```python
from build123d import *

# Parameters (mm, degrees)
F0_W      = 4.7625
F0_H      = 457.2
F1_DEPTH  = 609.6
F2_W      = 50.8
F2_H      = 4.7625
F3_DEPTH  = 609.6
F4_DEPTH  = 609.6
F5_W      = 25.4
F5_H      = 461.9625
F6_DEPTH  = 25.4
F8_DEPTH  = 25.4
F9_W      = 1637.8936
F9_H      = 25.4
F10_DEPTH = 25.4
F11_W     = 25.4
F11_H     = 433.81924
F12_DEPTH = 25.4
F13_DEPTH = 25.4
F14_W     = 25.4
F14_H     = 432.793116
F15_DEPTH = 25.4
F16_W     = 1636.5474
F16_H     = 25.4
F17_DEPTH = 25.4
F18_W     = 25.4
F18_H     = 609.6
F19_DEPTH = 25.4
F20_W     = 50.8
F20_H     = 453.430616
F21_DEPTH = 4.7625
F22_W     = 25.4
F22_H     = 457.2
F23_DEPTH = 4.7625


with BuildPart() as f1:
    # F0 (on Front) → F1 (new body)
    with BuildSketch(Plane.XZ):
        with Locations((-455.648437, -32.960023)):
            Rectangle(F0_W, F0_H)
        Polygon((-415.167187, -261.560023), (-453.267187, -261.560023), (-458.029687, -261.560023), (-458.029687, -266.322523), (-415.167187, -266.981946), align=None)
        Polygon((-408.817187, 151.189977), (-415.167187, -261.560023), (-415.167187, -266.981946), (-410.404687, -266.981946), (-404.044542, 146.427477), (-408.817187, 146.427477), align=None)
        Polygon((-403.971273, 151.189977), (-408.817187, 151.189977), (-408.817187, 146.427477), (-404.044542, 146.427477), align=None)
        Polygon((286.507813, 151.189977), (-403.971273, 151.189977), (-404.044542, 146.427477), (281.781948, 146.427477), (286.544448, 146.427477), align=None)
        Polygon((289.682813, -261.560023), (286.544448, 146.427477), (281.781948, 146.427477), (284.920313, -261.560023), align=None)
        Polygon((327.782813, -261.560023), (289.682813, -261.560023), (284.920313, -261.560023), (284.920313, -266.322523), (327.782813, -266.322523), align=None)
        Polygon((330.957813, 151.189977), (327.782813, -261.560023), (327.782813, -266.322523), (332.545172, -266.359156), (335.720454, 146.427477), (330.957813, 146.427477), align=None)
        Polygon((335.757089, 151.189977), (330.957813, 151.189977), (330.957813, 146.427477), (335.720454, 146.427477), align=None)
        Polygon((1021.520313, 151.189977), (335.757089, 151.189977), (335.720454, 146.427477), (1021.593582, 146.427477), align=None)
        Polygon((1026.282813, 151.189977), (1021.520313, 151.189977), (1021.593582, 146.427477), (1026.356082, 146.427477), align=None)
        Polygon((1026.356082, 146.427477), (1021.593582, 146.427477), (1027.870313, -261.560023), (1032.632813, -261.560023), align=None)
        Polygon((1032.632813, -261.560023), (1027.870313, -261.560023), (1027.870313, -266.322523), (1070.732813, -266.322523), (1070.732813, -261.560023), align=None)
        Polygon((1070.732813, 190.877477), (1070.732813, -261.560023), (1070.732813, -266.322523), (1075.495313, -266.322523), (1075.495313, 190.877477), align=None)
    extrude(amount=-F1_DEPTH)

    # F2 (on face) → F3 (join)
    with BuildSketch(Plane.XZ):
        with Locations((-483.429687, 193.258727)):
            Rectangle(F2_W, F2_H)
    extrude(amount=-F3_DEPTH)

    # F2 (on face) → F4 (join)
    with BuildSketch(Plane.XZ):
        with Locations((-483.429687, 193.258727)):
            Rectangle(F2_W, F2_H)
        with Locations((1100.895313, 188.496227)):
            Rectangle(F2_W, F2_H)
    extrude(amount=-F4_DEPTH)

    # F5 (on face) → F6 (join)
    with BuildSketch(Plane.XZ):
        with Locations((-496.129687, -40.103773)):
            Rectangle(F5_W, F5_H)
        with Locations((1113.595313, -44.866273)):
            Rectangle(F5_W, F5_H)
    extrude(amount=-F6_DEPTH)

    # F5 (on face) → F8 (join)
    with BuildSketch(Plane.XZ):
        with Locations((-496.129687, -40.103773)):
            Rectangle(F5_W, F5_H)
        with Locations((1113.595313, -44.866273)):
            Rectangle(F5_W, F5_H)
    extrude(amount=-F8_DEPTH)

    # F9 (on face) → F10 (join)
    with BuildSketch(Plane.XZ):
        with Locations((308.156171, -281.041763)):
            Rectangle(F9_W, F9_H)
    extrude(amount=-F10_DEPTH)

    # F11 (on face) → F12 (join)
    with BuildSketch(Plane.YZ.offset(1126.295313)):
        Polygon((609.6, 190.877477), (0, 190.877477), (0, 165.477477), (584.2, 165.477477), (609.6, 165.477477), align=None)
        with Locations((596.9, -51.432143)):
            Rectangle(F11_W, F11_H)
        Polygon((609.6, -293.741763), (609.6, -268.341763), (584.2, -268.341763), (25.4, -268.341763), (25.4, -293.741763), align=None)
    extrude(amount=-F12_DEPTH)

    # F11 (on face) → F13 (join)
    with BuildSketch(Plane.YZ.offset(1126.295313)):
        Polygon((609.6, 190.877477), (0, 190.877477), (0, 165.477477), (584.2, 165.477477), (609.6, 165.477477), align=None)
        with Locations((596.9, -51.432143)):
            Rectangle(F11_W, F11_H)
        Polygon((609.6, -293.741763), (609.6, -268.341763), (584.2, -268.341763), (25.4, -268.341763), (25.4, -293.741763), align=None)
    extrude(amount=-F13_DEPTH)

    # F14 (on face) → F15 (join)
    with BuildSketch(Plane(origin=(-508.829687, 0, 0), x_dir=(0, -1, 0), z_dir=(-1, 0, 0))):
        Polygon((-25.4, 165.477477), (-25.4, 190.877477), (-609.6, 190.877477), (-609.6, 165.477477), (-584.2, 165.477477), (-50.8, 165.477477), align=None)
        with Locations((-38.1, -50.919081)):
            Rectangle(F14_W, F14_H)
        with Locations((-596.9, -50.919081)):
            Rectangle(F14_W, F14_H)
        Polygon((-25.4, -292.715639), (-25.4, -267.315639), (-50.8, -267.315639), (-584.2, -267.315639), (-609.6, -267.315639), (-609.6, -292.715639), align=None)
    extrude(amount=-F15_DEPTH)

    # F16 (on face) → F17 (join)
    with BuildSketch(Plane(origin=(0, 0, -292.715639), x_dir=(1, 0, 0), z_dir=(0, 0, -1))):
        with Locations((309.444013, -596.9)):
            Rectangle(F16_W, F16_H)
    extrude(amount=-F17_DEPTH)

    # F18 (on face) → F19 (join)
    with BuildSketch(Plane(origin=(0, 0, -293.741763), x_dir=(1, 0, 0), z_dir=(0, 0, -1))):
        with Locations((307.752342, -304.8)):
            Rectangle(F18_W, F18_H)
    extrude(amount=-F19_DEPTH)

    # F20 (on face) → F21 (join)
    with BuildSketch(Plane(origin=(0, 609.6, 0), x_dir=(-1, 0, 0), z_dir=(0, 1, 0))):
        with Locations((-1100.895313, -40.600331)):
            Rectangle(F20_W, F20_H)
    extrude(amount=-F21_DEPTH)

    # F22 (on face) → F23 (join)
    with BuildSketch(Plane(origin=(0, 609.6, 0), x_dir=(-1, 0, 0), z_dir=(0, 1, 0))):
        with Locations((470.729687, -37.722523)):
            Rectangle(F22_W, F22_H)
    extrude(amount=-F23_DEPTH)


solid = f1.part
```
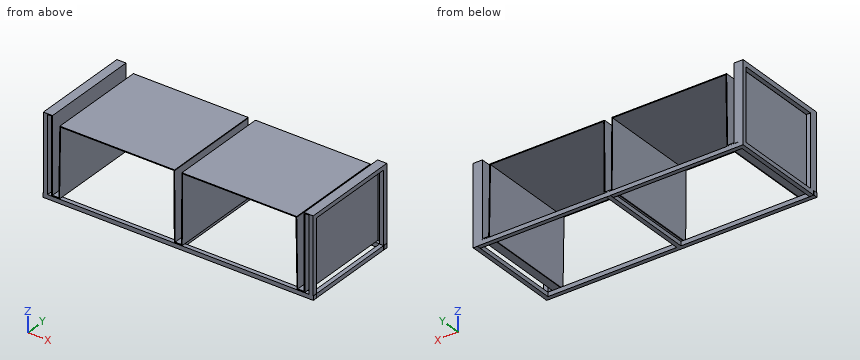
For this review, take the finished solid that the model builds, in its own axes (mm). Give positions to 0.01 mm unless a question says otherwise; leave off trailing zeros. Write each loop counter-clockwise with the first axis right and the second up, starting at its lowest first coordinate (ties: lowest second). Pieces come first, ordered by that corner, then holes.
Item 1: Take a section at A-A (x = 472). Give the boundary of the cut face in (y, z).
Item 2: Wall thickness on probe 1 along X at (y, z) = (373, 133.5); probe 2 along X at (y, z) = (448.5, -249); probe 3 along X at (y, z) = (559, 154): over which ranges is each line inside the solid? List them lowest first.
Item 3: Take a section at B-B (y = 198). Give the number of separate pieces and of enclosed holes in the cut face, and give its area (3 significant figures).
Item 4: Insertion check: P1, Ø7.5, axis at x = 1115.5, y = 419.5, coming from the +Z side; P2, Ø1.4, axis at y = 424.5, z = -264.5, coming from the -X side; P3, Ø7.5, axis at y = 434.5, z = -275.5, coming from the +X side. Each pin has a flat end and moves straight along its axis. Give the tip position at first contact, or say it passes through.
Established:
1. outline: (0, -293.74) - (25.4, -293.74) - (25.4, -268.34) - (0, -268.34) - close; (0, 146.43) - (609.6, 146.43) - (609.6, 151.19) - (0, 151.19) - close; (584.2, -292.72) - (609.6, -292.72) - (609.6, -267.32) - (584.2, -267.32) - close
2. probe 1: x = -458.03 to -453.27, -409.09 to -404.24, 281.88 to 286.64, 330.82 to 335.62, 1021.79 to 1026.55, 1070.73 to 1075.5
2. probe 2: x = -458.03 to -453.27, -414.97 to -410.13, 284.82 to 289.59, 327.88 to 332.68, 1027.68 to 1032.44, 1070.73 to 1075.5
2. probe 3: x = -458.03 to -453.27, 1070.73 to 1075.5
3. separate pieces: 4
3. enclosed holes: 0
3. area: 23,100 mm2
4. P1: stops at z = 190.88
4. P2: stops at x = -458.03
4. P3: stops at x = 1126.3
